Read the model definition and answer for the solid it produces. Units are mm, in the model's axes. Give positions to 0.01 mm unless a question says otherwise; leave off trailing zeros. Write each loop counter-clockwise with the first axis right and the second up, starting at its lowest first coordinate (ties: lowest second). Pieces come first, ordered by that corner, then holes. Notation, with made-up numbers: M -34.5,56 L 2.5,56 A22 cw 2.5,66 Z; hole C 16.5,35 d2. An arc over 180 degrees is marked long. Use a Markdown table: item, result. Add a question column.
Item 1: Consider probe 1 along Y at (x, z) = (7.75, 2.55); probe 2 along Y at (x, z) = (-0.5, 4.3); probe 3 along Y at (x, z) = (22.5, 4.4). Determine where each line is inside the solid, lowest interval first. Write a range as [from, to].
Item 2: A cutting plane is placed at C-C on z = 2. Count the separate pieces of the cut face and the enclosed holes in it, then the cut area to 3 significant figures.
Item 3: A cutting plane is placed at A-A on y = 38. Determine the outline of the cut face in (x, z), then the cut area to 4 significant figures.
Item 4: The mould has two halves that part along X. Classify faces 1 (the flat face through (-16, 8, 0)), 2 (the flat face through (-60, 8, 2)), 3 (the cylindrical face through (10.61, -34.11, 2.46)): pulls with the +X half, pulls with the -X half, needs draft (parallel to the pull), parting line crosses it, or undercut.
Item 5: A cutting plane is placed at B-B on x = 11.5. Determine the outline of the cut face in (y, z), then the cut area to 4 significant figures.
from build123d import *

# Parameters (mm, degrees)
SKETCH_2_R          = 1.6
SKETCH_2_R_2        = 7
EXTRUDE_1_DEPTH     = 5
SKETCH_4_R          = 3.004319303
CUT_EXTRUDE_2_DEPTH = 10
SKETCH_5_R          = 1.65
SKETCH_5_R_2        = 1.5
CUT_EXTRUDE_3_DEPTH = 10


with BuildPart() as part:
    # Эскиз2 → Бобышка-Вытянуть1 (new body)
    with BuildSketch(Plane.XY):
        Polygon((-25, 62), (-60, 62), (-60, -48), (-25, -48), (30, -48), (30, 62), align=None)
        with Locations((-15.5, 0)):
            Circle(SKETCH_2_R, mode=Mode.SUBTRACT)
        with Locations((-7.75, 13.423393759)):
            Circle(SKETCH_2_R, mode=Mode.SUBTRACT)
        with Locations((7.75, 13.423393759)):
            Circle(SKETCH_2_R, mode=Mode.SUBTRACT)
        with Locations((15.5, 0)):
            Circle(SKETCH_2_R, mode=Mode.SUBTRACT)
        with Locations((7.75, -13.423393759)):
            Circle(SKETCH_2_R, mode=Mode.SUBTRACT)
        with Locations((-7.75, -13.423393759)):
            Circle(SKETCH_2_R, mode=Mode.SUBTRACT)
        with Locations((0, 7)):
            Circle(SKETCH_2_R_2, mode=Mode.SUBTRACT)
    extrude(amount=EXTRUDE_1_DEPTH)

    # Эскиз4 → Вырез-Вытянуть2 (cut)
    with BuildSketch(Plane.XY.offset(5)):
        with Locations((22.80785145, 10.989617997)):
            Circle(SKETCH_4_R)
    extrude(amount=-CUT_EXTRUDE_2_DEPTH, mode=Mode.SUBTRACT)

    # Эскиз5 → Вырез-Вытянуть3 (cut)
    with BuildSketch(Plane(origin=(0, 0, 0), x_dir=(-1, 0, 0), z_dir=(0, 0, -1))):
        with Locations((-17.551724138, 51)):
            Circle(SKETCH_5_R)
        with Locations((-5.448275862, 38)):
            Circle(SKETCH_5_R)
        with Locations((32.234685073, -33.82)):
            Circle(SKETCH_5_R_2)
        with Locations((47.765314927, -9.82)):
            Circle(SKETCH_5_R_2)
        with Locations((-11.5, -35.5)):
            Circle(SKETCH_5_R)
    extrude(amount=-CUT_EXTRUDE_3_DEPTH, mode=Mode.SUBTRACT)


solid = part.part
Filled in:
| question | item | result |
|---|---|---|
| 1 | probe 1 | [-48, -15.02], [-11.82, 11.82], [15.02, 62] |
| 1 | probe 2 | [-48, 0.02], [13.98, 62] |
| 1 | probe 3 | [-48, 8], [13.98, 62] |
| 2 | separate pieces | 1 |
| 2 | enclosed holes | 13 |
| 2 | area | 9,630 mm² |
| 3 | outline | M -60,0 L 3.8,0 L 3.8,5 L -60,5 Z; M 7.1,0 L 30,0 L 30,5 L 7.1,5 Z |
| 3 | area | 433.5 mm² |
| 4 | face 1 | needs draft |
| 4 | face 2 | pulls with the -X half |
| 4 | face 3 | undercut |
| 5 | outline | M -48,0 L -37.15,0 L -37.15,5 L -48,5 Z; M -33.85,0 L 62,0 L 62,5 L -33.85,5 Z |
| 5 | area | 533.5 mm² |
